from build123d import *

# Parameters (mm, degrees)
BOSS_EXTRUDE1_DEPTH        = 38.1
BOSS_EXTRUDE2_DEPTH        = 9.525
SKETCH3_R                  = 16.002
BOSS_EXTRUDE3_DEPTH        = 4.572
BOSS_EXTRUDE4_DEPTH        = 4.7625
FILLET1_R                  = 15.875
FILLET2_R                  = 12.7
F_1_4_0_5_DIAMETER_HOLE1_D = 12.7
F_1_4_0_5_DIAMETER_HOLE2_D = 12.7


with BuildPart() as part:
    # Sketch1 → Boss-Extrude1 (new body, symmetric)
    with BuildSketch(Plane(origin=(0, 0, 0), x_dir=(0, 0, -1), z_dir=(1, 0, 0))):
        with BuildLine():
            Line((0, 0), (-37.084, 0))
            Line((-37.084, 0), (-37.084, -9.525))
            Line((-37.084, -9.525), (2.54, -9.525))
            Line((2.54, -9.525), (2.54, -2.54))
            ThreePointArc((2.54, -2.54), (0.743948776, -1.796051224), (0, 0))
        make_face()
    extrude(amount=BOSS_EXTRUDE1_DEPTH, both=True)

    # Sketch2 → Boss-Extrude2 (add)
    with BuildSketch(Plane.XY):
        with BuildLine():
            Line((-16.002, 0), (16.002, 0))
            Line((16.002, 0), (16.002, 53.975))
            ThreePointArc((16.002, 53.975), (0, 69.977), (-16.002, 53.975))
            Line((-16.002, 53.975), (-16.002, 0))
        make_face()
    extrude(amount=BOSS_EXTRUDE2_DEPTH)

    # Sketch3 → Boss-Extrude3 (add)
    with BuildSketch(Plane(origin=(0, 0, 0), x_dir=(-1, 0, 0), z_dir=(0, 0, -1))):
        with Locations((0, 53.975)):
            Circle(SKETCH3_R)
    extrude(amount=BOSS_EXTRUDE3_DEPTH)

    # Sketch4 → Boss-Extrude4 (add, symmetric)
    with BuildSketch(Plane(origin=(0, 0, 0), x_dir=(0, 0, -1), z_dir=(1, 0, 0))):
        Polygon((-9.525, 41.275), (-37.084, 0), (-9.525, 0), align=None)
    extrude(amount=BOSS_EXTRUDE4_DEPTH, both=True)

    # Fillet1
    fillet1_edges = [part.edges().sort_by_distance(p)[0] for p in [
        (-16.002, 0, 4.7625),
        (16.002, 0, 4.7625),
    ]]
    fillet(fillet1_edges, radius=FILLET1_R)

    # Fillet2
    fillet2_edges = [part.edges().sort_by_distance(p)[0] for p in [
        (38.1, -4.7625, 37.084),
        (-38.1, -4.7625, 37.084),
    ]]
    fillet(fillet2_edges, radius=FILLET2_R)

    # 1/4 (0.5) Diameter Hole1 (through all)
    with Locations(Plane(origin=(0, 0, 0), x_dir=(1, 0, 0), z_dir=(0, 1, 0))):
        with Locations((-25.4, -24.384), (25.4, -24.384)):
            Hole(F_1_4_0_5_DIAMETER_HOLE1_D / 2)

    # 1/4 (0.5) Diameter Hole2 (through all)
    with Locations(Plane.XY.offset(9.525)):
        with Locations((0, 53.975)):
            Hole(F_1_4_0_5_DIAMETER_HOLE2_D / 2)


solid = part.part
Geometry: final body of the model. Coordinates: model frame, mm. A direction names the side the tool comes from. Give positions to 0.01 mm unless a question says otherwise; leave off trailing zeros. Write each loop counter-clockwise with the first axis right and the second up, starting at its lowest first coordinate (ties: lowest second). Pieces come first, ordered by that corner, then holes. Notation, with made-up numbers: M -15,65 L -6,65 A25 cw -6,97 Z; hole C -29,70.5 d9. An arc over 180 degrees is marked long. Answer in a Markdown table with one row per item. Add a question column.
(1) Section B-B on z = 25.5. Return loops of the section in (x, y) (1 decimal), and give its area (3 significant figures).
(2) Section A-A on x = 0. Return loops of the section in (y, z) (3 decimals).
(3) Section C-C on y = 51. Return loops of the section in (x, z) (3 decimals).
(4) First-contact query: pin 1 (8.5 mm diameter, centred on y = 31, z = 18.5, fed in from -X); pin 2 (10.5 mm diameter, centred on y = 31, z = 6.5, fed in from -X); pin 3 (10 mm diameter, centred on y = 18.5, z = 13, fed in from +X). Flat tips, straight axial feed; report the tip coordinate or a pass-through.
(5) Mould query, pull axis Z, two halves, no side actions, for faces 1 (the cylindrical face through (0.533, -1.816, -0.764)), 2 (the cylindrical face through (26.23, -4.83, 18.09)), 3 (the cylindrical face through (-24.57, -4.83, 18.09)), 4 (the flat face through (16.002, 35, 5)). Classes: +Z half, -Z half, draft (parallel to the pull), parting line (faces both ways), or undercut.
(6) Ray query, line 1 (Z direction, x = -25.4, y = -7); line 2 (Y direction, x = 0, z = 4) (3 decimals); line 3 (Y direction, x = 0, z = -0.5) (3 decimals). Return the intervals inside material, ascending.
(7) Reachability of faces 5 (the flat face through (-21, 0, 18)), 6 (the flat face through (-16.002, 35, 5)), 7 (the flat face through (1, -6, -2.54)) from +Z, -Z, +X, -X, +Y, -Y: full face, straight path, thin tool, end or side. Return the list, or none.
(8) Section D-D on z = 7.5. Return loops of the section in (x, y) (3 decimals), and give its area (3 significant figures).
Result set:
| question | item | result |
|---|---|---|
| 1 | outline | M -38.1,-9.5 L -31.7,-9.5 L -31.7,0 L -38.1,0 Z; M -19.1,-9.5 L 19.1,-9.5 L 19.1,0 L 4.8,0 L 4.8,17.3 L -4.8,17.3 L -4.8,0 L -19.1,0 Z; M 31.7,-9.5 L 38.1,-9.5 L 38.1,0 L 31.7,0 Z |
| 1 | area | 652 mm^2 |
| 2 | outline | M -9.525,-2.54 L -2.54,-2.54 A2.54 cw 0,0 L 37.973,0 L 37.973,-4.572 L 47.625,-4.572 L 47.625,9.525 L 41.275,9.525 L 0,37.084 L -9.525,37.084 Z; M 60.325,-4.572 L 69.977,-4.572 L 69.977,9.525 L 60.325,9.525 Z |
| 3 | outline | M -16.002,0 L -15.723,0 L -15.723,-4.572 L -5.61,-4.572 L -5.61,9.525 L -16.002,9.525 Z; M 5.61,-4.572 L 15.723,-4.572 L 15.723,0 L 16.002,0 L 16.002,9.525 L 5.61,9.525 Z |
| 4 | pin 1 | stops at x = -4.76 |
| 4 | pin 2 | stops at x = -16 |
| 4 | pin 3 | stops at x = 16.03 |
| 5 | face 1 | -Z half |
| 5 | face 2 | undercut |
| 5 | face 3 | undercut |
| 5 | face 4 | draft |
| 6 | line 1 | z = -2.54 to 18.03, 30.73 to 37.08 |
| 6 | line 2 | y = -9.525 to 47.625, 60.325 to 69.977 |
| 6 | line 3 | y = -9.525 to -1.513, 37.973 to 47.625, 60.325 to 69.977 |
| 7 | face 5 | +Z, -X, +Y |
| 7 | face 6 | +Z, -Z, -X, +Y |
| 7 | face 7 | -Z, +X, -X, -Y |
| 8 | outline | M -38.1,-9.525 L 38.1,-9.525 L 38.1,0 L 31.877,0 A15.875 cw 16.002,15.875 L 16.002,53.975 A16.002 ccw -16.002,53.975 L -16.002,15.875 A15.875 cw -31.877,0 L -38.1,0 Z; hole C 0,53.975 d12.7 |
| 8 | area | 2,840 mm^2 |
